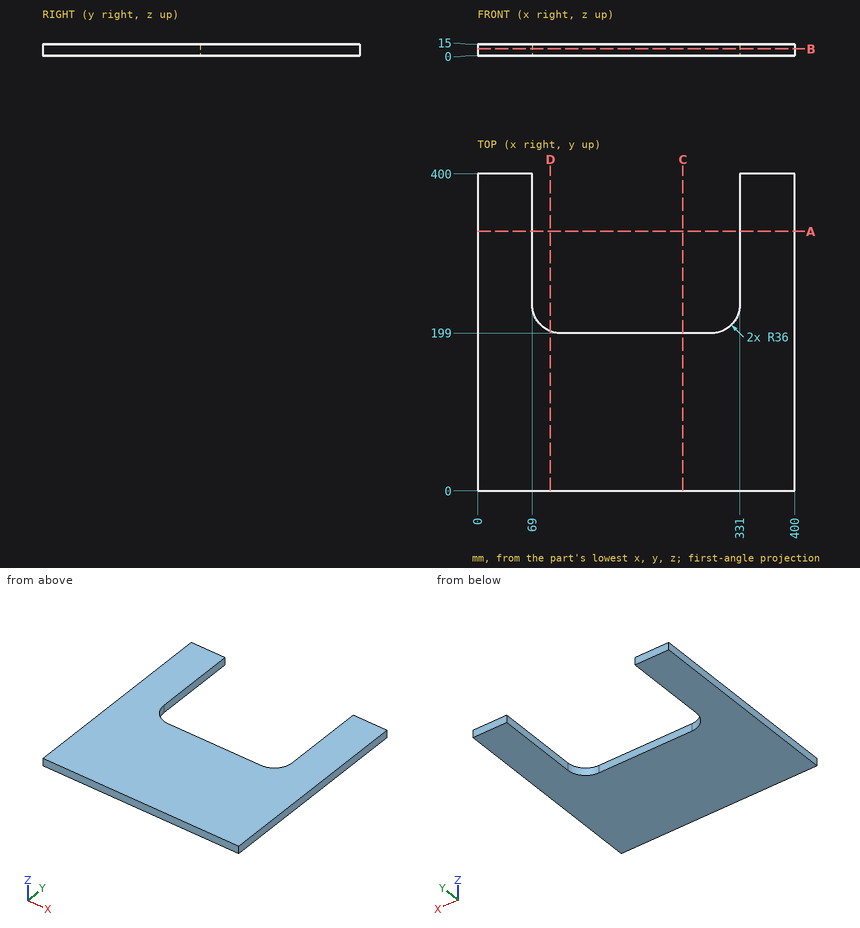
Job drawing, mm, ordinate dimensions from the low corner. One solid piece. Coordinates: 2 decimals unless noted, no trailing zeros. Write each loop counter-clockwise with the first axis right and the second up, starting at its lowest first coordinate (ties: lowest second). Pieces come first, ordered by that corner, then holes. Notation, with made-up numbers: M -35.5,4 L -29.5,4 A25 cw -29.5,42 Z; hole C 88,-8.75 d7. An arc over 180 degrees is marked long. Answer as a JSON object with one key per item and string values. Group by question number.
1) Saw through at A-A (y = 327.5). Write the cut outline in (x, z).
2) Saw through at C-C (x = 259). Write the cut outline in (y, z).
3) Saw through at B-B (z = 9). Write the cut outline in (x, y).
4) Saw through at D-D (x = 92). Write the cut outline in (y, z).
5) Pin check, flat tip, straight feed: pin 1 Ø4.5 at (x, z) = (202, 4) entering from +Y. Stop position of the tip, or through.
6) Wall check: line 1 (X direction, y = 357.5, z = 1.25); line 2 (Y direction, x = 253, z = 1.25); line 3 (Y direction, x = 297.5, z = 2.75). Give the ranges that are in metal, low to high. Write a range as from..to.
Values follow:
{
 "1": {"outline": "M 0,0 L 69,0 L 69,15 L 0,15 Z; M 331,0 L 400,0 L 400,15 L 331,15 Z"},
 "2": {"outline": "M 0,0 L 199,0 L 199,15 L 0,15 Z"},
 "3": {"outline": "M 0,0 L 400,0 L 400,400 L 331,400 L 331,235 A36 cw 295,199 L 105,199 A36 cw 69,235 L 69,400 L 0,400 Z"},
 "4": {"outline": "M 0,0 L 201.43,0 L 201.43,15 L 0,15 Z"},
 "5": {"pin 1": "stops at y = 199"},
 "6": {"line 1": "x = 0..69, 331..400", "line 2": "y = 0..199", "line 3": "y = 0..199.09"}
}
